from build123d import *

# Parameters (mm, degrees)
SKETCH1_R           = 5.75
BOSS_EXTRUDE1_DEPTH = 15
CUT_EXTRUDE3_DEPTH  = 8
SKETCH7_W           = 3.7
SKETCH7_H           = 5.5
CUT_EXTRUDE4_DEPTH  = 6.5


with BuildPart() as part:
    # Sketch1 → Boss-Extrude1 (new body)
    with BuildSketch(Plane(origin=(0, 0, 0), x_dir=(1, 0, 0), z_dir=(0, 1, 0))):
        with Locations(Location((0, 0, 0), (0, 0, 270))):
            Circle(SKETCH1_R)
    extrude(amount=BOSS_EXTRUDE1_DEPTH)

    # Sketch6 → Cut-Extrude3 (cut)
    with BuildSketch(Plane(origin=(0, 15, 0), x_dir=(1, 0, 0), z_dir=(0, 1, 0))):
        with BuildLine():
            Line((0.41, 2.964671599), (0.41, -2.964671599))
            ThreePointArc((0.41, -2.964671599), (3.374671599, 0), (0.41, 2.964671599))
        make_face()
        with BuildLine():
            Line((-0.416408681, 2.965564682), (-0.416408681, -2.965564682))
            ThreePointArc((-0.416408681, -2.965564682), (-3.381973363, 0), (-0.416408681, 2.965564682))
        make_face()
    extrude(amount=-CUT_EXTRUDE3_DEPTH, mode=Mode.SUBTRACT)

    # Sketch7 → Cut-Extrude4 (cut)
    with BuildSketch(Plane(origin=(0, 0, 0), x_dir=(1, 0, 0), z_dir=(0, 1, 0))):
        Rectangle(SKETCH7_W, SKETCH7_H)
    extrude(amount=CUT_EXTRUDE4_DEPTH, mode=Mode.SUBTRACT)


solid = part.part
Check sheet for the modelled part. Datum: model origin and axes. Units: mm. A direction names the side the tool comes from. Round coordinates to 2 decimals unless told otherwise and drop trailing zeros. Order: outer loops, then holes, each group sorted by start corner. A loop starts at its lowest first (then second) coordinate and runs counter-clockwise, first axis right, second up. Notation, with made-up numbers: M -13.75,74 L 38.25,74 A20 cw 38.25,103 Z; hole C 63,9 d6. An arc over 180 degrees is marked long. One line per item, written item: value. Start each with the question number.
1. Section check B-B on y = 3.25. Enter the section's corners in (x, z).
2. Scan lines: line 1 along X through (y, z) = (9.75, 0); line 2 along X through (y, z) = (13, -2); line 3 along Y through (x, z) = (-0.25, 2.5). Record each from-to range of solid material in increasing order.
3. Section check D-D on x = 0. Enter the section's corners in (y, z).
4. Section check C-C on z = 0. Enter the section's corners in (x, y).
5. Release check for a two-part mould opening along Z. For faces 4 (the cylindrical face through (4.85, 7.4, 3.09)), 5 (the flat face through (0, 6.5, 0)), 6 (the flat face through (-2.5, 0, -0.1)) record: released by +Z, released by -Z, zero draft, split by the parting line, or undercut.
6. Gauge pin test, flat ends, axial feed: P1, Ø3, axis at y = 13.5, z = 3, coming from the -X side; P2, Ø0.9, axis at x = -2, z = 1.5, coming from the +Y side; P3, Ø4, axis at y = 12.5, z = -2.5, coming from the -X side. Record the tip position at first contact, or that the pin passes through.
7. Section check A-A on y = 14. Enter the section's corners in (x, z).
8. Access from +Z, -Z, +X, -X, +Y, -Y to the whole of each face (thin tool, end or side, straight path). Record for faces 1 (the cylindrical face through (-3.38, 11.06, 0.07)), 2 (the flat face through (0, 15, 0)), 3 (the flat face through (-1.85, 3, 0)).
Results found:
1. outline: C 0,0 d11.5; hole M -1.85,-2.75 L 1.85,-2.75 L 1.85,2.75 L -1.85,2.75 Z
2. line 1: -5.75 to -3.38, -0.42 to 0.41, 3.37 to 5.75
2. line 2: -5.39 to -2.61, -0.42 to 0.41, 2.6 to 5.39
2. line 3: 6.5 to 15
3. outline: M 0,-5.75 L 15,-5.75 L 15,5.75 L 0,5.75 L 0,2.75 L 6.5,2.75 L 6.5,-2.75 L 0,-2.75 Z
4. outline: M -5.75,0 L -1.85,0 L -1.85,6.5 L 1.85,6.5 L 1.85,0 L 5.75,0 L 5.75,15 L 3.37,15 L 3.37,7 L 0.41,7 L 0.41,15 L -0.42,15 L -0.42,7 L -3.38,7 L -3.38,15 L -5.75,15 Z
5. face 4: split by the parting line
5. face 5: undercut
5. face 6: zero draft
6. P1: x = -5.55
6. P2: y = 7
6. P3: x = -5.73
7. outline: C 0,0 d11.5; hole M -0.42,-2.97 L -0.42,2.97 A2.97 ccw Z; hole M 0.41,-2.96 A2.96 ccw 0.41,2.96 Z
8. face 1: +Y
8. face 2: +Z, -Z, +X, -X, +Y
8. face 3: -Y
